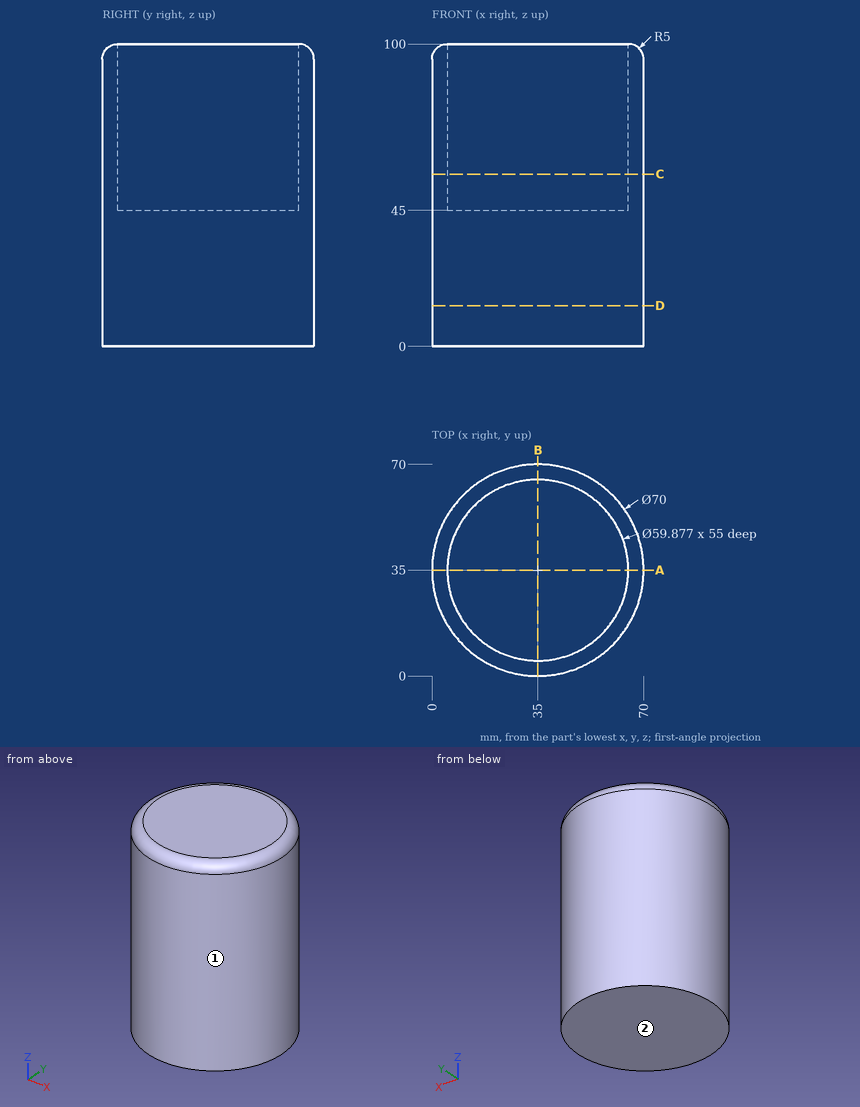
Could you check a few things on this drawing? It's one solid part, dimensions in mm from its lowest x, y, z. Coordinates: 2 decimals unless noted, no trailing zeros. Loops run counter-clockwise (first coordinate to the right, second up) from the corner with the lowest first, then second, coordinate; pieces in that order, holes last. Notation, with made-up numbers: (82, 70.5) - (113, 70.5) arc R22 cw to (113, 96.5) - close; hole circle Ø1 at (-7.5, 72.5). An arc over 180 degrees is marked (long way). Answer as a JSON object with one key per item and string values. Group by question number.
Item 1: If we section it at D-D (z = 13.5): List the corners of the cut face in (x, y) for me, plus the area to 3 significant figures.
Item 2: If we section it at C-C (z = 57): List the corners of the cut face in (x, y) for me.
Item 3: If we mould it in two halves opening along X, with no side actions, what happens to the marked faces 1 and 2? For each: released by +X, released by -X, zero draft, split by the parting line, or undercut.
Item 4: If I drill on L1, parallel to Y at x = 35, z = 69; L2, parallel to Z at x = 25, y = 28; L3, parallel to Y at x = 11.5, z = 59, over which ranges is the centre line in solid material (lowest first)? Write a range as from..to.
Item 5: For pin 1 (3 mm diameter, centred on y = 7, z = 16.5, fed in from -X); pin 2 (1 mm diameter, centred on x = 20, z = 35.5, fed in from +Y) (1 decimal); pin 3 (3 mm diameter, centred on y = 11, z = 37, fed in from +X), each with a flat end and sliding along its axis, tell me the tip position at first contact or that it passes through.
Item 6: If we section it at A-A (y = 35): List the corners of the cut face in (x, z) for me, plus the area to 3 significant figures.
Returned:
{
 "1": {"outline": "circle Ø70 at (35, 35)", "area": "3,850 mm²"},
 "2": {"outline": "circle Ø70 at (35, 35); hole circle Ø59.88 at (35, 35)"},
 "3": {"face 1": "split by the parting line", "face 2": "zero draft"},
 "4": {"L1": "y = 0..5.06, 64.94..70", "L2": "z = 0..45", "L3": "y = 9.06..16.45, 53.55..60.94"},
 "5": {"pin 1": "stops at x = 12.14", "pin 2": "stops at y = 66.9", "pin 3": "stops at x = 61.81"},
 "6": {"outline": "(0, 0) - (70, 0) - (70, 95) arc R5 ccw to (65, 100) - (64.94, 100) - (64.94, 45) - (5.06, 45) - (5.06, 100) - (5, 100) arc R5 ccw to (0, 95) - close", "area": "3,700 mm²"}
}
